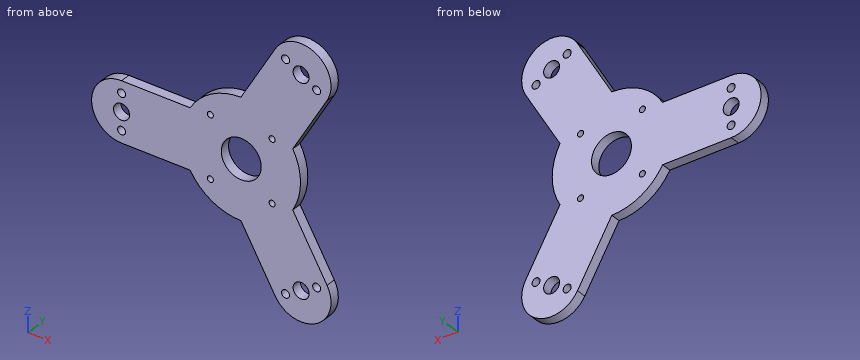
Autodesk Inventor part; units mm, degrees
ref_plane "YZ Plane" through (0, 0, 0) normal (1, 0, 0) x (0, 1, 0)
ref_plane "XZ Plane" through (0, 0, 0) normal (0, 1, 0) x (-1, 0, 0)
ref_plane "XY Plane" through (0, 0, 0) normal (0, 0, 1) x (1, 0, 0)
sketch "Sketch1" plane through (0, 0, 0) normal (0, 1, 0) x (-1, 0, 0)
  circle A0 centre (0, 0) radius 60
  circle A1 centre (60, 0) radius 4
  circle A2 centre (-30, 51.9615) radius 4
  circle A3 centre (-30, -51.9615) radius 4
  circle A4 centre (-30, 51.9615) radius 15
  circle A5 centre (-30, -51.9615) radius 15
  circle A6 centre (60, 0) radius 15
  line L0 (21, -21) -> (-21, -21)
  line L1 (-21, -21) -> (-21, 21)
  line L2 (-21, 21) -> (21, 21)
  line L3 (21, 21) -> (21, -21)
  line L4 (21, -21) -> (-21, 21) construction
  line L5 (-21, -21) -> (21, 21) construction
  line L6 (67.5, 12.9904) -> (-22.5, 64.9519)
  line L7 (67.5, -12.9904) -> (-22.5, -64.9519)
  line L8 (-45, 51.9615) -> (-45, -51.9615)
  circle A7 centre (0, 0) radius 10
  line L9 (67.5, 12.9904) -> (21, 39.8372)
  line L10 (60, 15) -> (25.632, 15)
  line L11 (60, -15) -> (25.632, -15)
  circle A8 centre (0, 0) radius 29.6985
  circle A9 centre (28.3546, 20) radius 5
  circle A10 centre (28.3546, -20) radius 5
  circle A11 centre (-31.4978, 14.5558) radius 5
  line L12 (-42.9904, 44.4615) -> (-25.8064, 14.698)
  line L13 (-17.0096, 59.4615) -> (0.1744, 29.698)
  circle A12 centre (3.1432, 34.5558) radius 5
  circle A13 centre (3.1432, -34.5558) radius 5
  line L14 (-17.0096, -59.4615) -> (0.1744, -29.698)
  line L15 (-42.9904, -44.4615) -> (-25.8064, -14.698)
  circle A14 centre (-31.4978, -14.5558) radius 5
  point P0 (16, -16)
  point P1 (16, 16)
  point P2 (-16, 16)
  point P3 (-16, -16)
  point P4 (-16.174, 57.7789)
  point P5 (-41.951, 42.8966)
  point P6 (-42.0378, 42.8115)
  point P7 (-25.8064, 14.698)
  point P8 (-25.8064, -14.698)
  point P9 (-42.0378, -42.8115)
  point P10 (-41.951, -42.8966)
  point P11 (-16.174, -57.7789)
  point P12 (-16.057, -57.8115)
  point P13 (58.0948, -15)
  point P14 (58.125, -14.8824)
  point P15 (58.125, 14.8824)
  point P16 (58.0948, 15)
  point P17 (-16.057, 57.8115)
  dimension "d0" = 120
  dimension "d2" = 8
  dimension "d5" = 360
  dimension "d7" = 30
  dimension "d8" = 30
  dimension "d9" = 30
  dimension "d10" = 42
  dimension "d11" = 42
  dimension "d12" = 20
  dimension "d13" = 32
  dimension "d14" = 16
  dimension "d15" = 16
  dimension "d16" = 32
  dimension "d17" = 10
  dimension "d18" = 10
  dimension "d21" = 360
extrude "Extrusion1" add sketch "Sketch1" along normal blind 5 contours A1 A0 A6 | A0 A6 A1 | A6 A0 L11 A8 L10 | A0 L10 A6 | A6 L11 A0 | A8 L3 | L13 A8 L12 A0 A4 | A0 A4 L13 | A4 A0 A2 | L3 L0 L1 L2 | L2 A8 | L14 A5 A0 | A0 A5 L15 A8 L14 | A5 A0 A3 | A8 L0 | A4 A0 A2 | L1 A8 | A0 A3 A5 | A4 A0 L12 | L15 A0 A5
sketch "Sketch2" plane through (0, 5, 0) normal (0, 1, 0) x (1, 0, 0)
  point P0 (0, 0)
  point P1 (-15.5, -15.5)
  point P2 (-15.5, 15.5)
  point P3 (15.5, -15.5)
  point P4 (15.5, 15.5)
  dimension "d25" = 31
  dimension "d26" = 31
  dimension "d27" = 15.5
  dimension "d28" = 15.5
hole "Hole1" at (-15.5, 5, 15.5) at (-15.5, 5, -15.5) at (15.5, 5, 15.5) at (15.5, 5, -15.5) direction (0, -1, 0) diameter 3.05 end through all
sketch "Sketch3" plane through (0, 5, 0) normal (0, 1, 0) x (1, 0, 0)
  circle A0 centre (-60, 0) radius 4
  point P0 (0, 0)
  point P1 (-60, -9)
  point P2 (-60, 9)
  dimension "d36" = 9
  dimension "d37" = 18
hole "Hole2" at (-60, 5, 9) at (-60, 5, -9) direction (0, -1, 0) diameter 4 end through all
pattern_circular "Circular Pattern1" count 3 over 360 about axis through (0, 0, 0) along (0, 1, 0) of "Hole2"
properties part number "De_Duoi" material "Aluminum 6061"
Input: part model. Units: mm. Frame: model coordinates. Coordinates: 2 decimals unless noted, no trailing zeros. Loops run counter-clockwise (first coordinate to the right, second up) from the corner with the lowest first, then second, coordinate; pieces in that order, holes last. Notation, with made-up numbers: M 63,33.5 L 93,33.5 A15 cw 93,59.5 Z; hole C 23.25,43 d1. An arc over 180 degrees is marked long. Use a Markdown table: item, result. Add a question column.
1) Section A-A, the plane x = 7.5. Return the cut outline in (y, z), plus the area to 3 significant figures.
2) Line query: L1, parallel to Z at x = -60, y = 1.85; L2, parallel to X at y = 1.15, z = 0.5; L3, parallel to Z at x = 30, y = 3.4. Output: solid intervals per line, ascending. Write a range as from..to.
3) Section D-D, the plane z = -20.5. Return the cut outline in (x, y).
4) Section C-C, the plane x = -54. Return the cut outline in (y, z).
5) Pin query (flat end, axial travel): P1, Ø2, axis at y = 0.5, z = -33, coming from the +X side; P2, Ø3, axis at x = 22.21, z = 56.46, coming from the -Y side; P3, Ø4, axis at x = 15.5, z = -15.5, coming from the -Y side; P4, Ø1.5, axis at x = -35.5, y = 3, coming from the -Z side. Return the tip coordinate at first contact, or that it passes through.
Answer below:
| question | item | result |
|---|---|---|
| 1 | outline | M 0,-42.99 L 5,-42.99 L 5,-6.61 L 0,-6.61 Z; M 0,6.61 L 5,6.61 L 5,42.99 L 0,42.99 Z |
| 1 | area | 364 mm2 |
| 2 | L1 | -15..-11, -7..-4, 4..7, 11..15 |
| 2 | L2 | -74.99..-63.97, -56.03..-9.99, 9.99..29.69 |
| 2 | L3 | -66.96..-55.96, -47.96..-21.96, 21.96..47.96, 55.96..66.96 |
| 3 | outline | M -21.49,0 L 29.16,0 L 29.16,5 L -21.49,5 Z |
| 4 | outline | M 0,-15 L 5,-15 L 5,15 L 0,15 Z |
| 5 | P1 | x = 36.95 |
| 5 | P2 | through |
| 5 | P3 | y = 0 |
| 5 | P4 | z = -15 |
